```python
from build123d import *

# Parameters (mm, degrees)
SKETCH1_W                                = 68.4872
SKETCH1_H                                = 20.55
BOSS_EXTRUDE1_DEPTH                      = 28.732
SKETCH2_W                                = 55.7872
SKETCH2_H                                = 18.207
CUT_EXTRUDE1_DEPTH                       = 21.55
F_2_5_2_5_DIAMETER_HOLE1_AT_2_COUNT      = 2
F_2_5_2_5_DIAMETER_HOLE1_AT_2_PITCH      = 62.1372
F_3_2_3_2_DIAMETER_HOLE1_AT_2_COUNT      = 2
F_3_2_3_2_DIAMETER_HOLE1_AT_2_PITCH      = 62.1372
F_5_16_0_3125_DIAMETER_HOLE1_D           = 7.9375
F_5_16_0_3125_DIAMETER_HOLE1_CSINK_D     = 9.2075
F_5_16_0_3125_DIAMETER_HOLE1_CSINK_ANGLE = 90
F_1_8_0_125_DIAMETER_HOLE1_D             = 3.175
F_1_8_0_125_DIAMETER_HOLE1_DEPTH         = 9.53
F_1_8_0_125_DIAMETER_HOLE1_CSINK_D       = 3.81
F_1_8_0_125_DIAMETER_HOLE1_CSINK_ANGLE   = 90
F_1_8_0_125_DIAMETER_HOLE1_TIP           = 0.953866233


with BuildPart() as part:
    # Sketch1 → Boss-Extrude1 (new body)
    with BuildSketch(Plane(origin=(0, 0, 0), x_dir=(1, 0, 0), z_dir=(0, 1, 0))):
        with Locations((0, 10.275)):
            Rectangle(SKETCH1_W, SKETCH1_H)
    extrude(amount=BOSS_EXTRUDE1_DEPTH)

    # Sketch2 → Cut-Extrude1 (cut, through all)
    with BuildSketch(Plane.XY):
        with Locations((0, 19.6285)):
            Rectangle(SKETCH2_W, SKETCH2_H)
    extrude(amount=-CUT_EXTRUDE1_DEPTH, mode=Mode.SUBTRACT)

    # Sketch5 → Ø2.5 (2.5) Diameter Hole1 (revolve, cut)
    with BuildSketch(Plane(origin=(-31.0686, 21.5, 0), x_dir=(0, -1, 0), z_dir=(1, 0, 0))):
        Polygon((0, 0), (0, 20.55), (1.375, 20.55), (1.25, 20.425), (1.25, 0.125), (1.375, 0), align=None)
    f_2_5_2_5_diameter_hole1 = revolve(axis=Axis((-31.0686, 21.5, 6.35), (0, 0, -1)), mode=Mode.SUBTRACT)

    # Ø2.5 (2.5) Diameter Hole1 at 2: Ø2.5 (2.5) Diameter Hole1 ×2
    with Locations(*[(i * F_2_5_2_5_DIAMETER_HOLE1_AT_2_PITCH, 0, 0) for i in range(1, F_2_5_2_5_DIAMETER_HOLE1_AT_2_COUNT)]):
        add(f_2_5_2_5_diameter_hole1, mode=Mode.SUBTRACT)

    # Sketch8 → Ø3.2 (3.2) Diameter Hole1 (revolve, cut)
    with BuildSketch(Plane(origin=(-31.0686, 10.5, 0), x_dir=(0, -1, 0), z_dir=(1, 0, 0))):
        Polygon((0, 0), (0, 20.55), (1.75, 20.55), (1.6, 20.4), (1.6, 0.15), (1.75, 0), align=None)
    f_3_2_3_2_diameter_hole1 = revolve(axis=Axis((-31.0686, 10.5, 6.35), (0, 0, -1)), mode=Mode.SUBTRACT)

    # Ø3.2 (3.2) Diameter Hole1 at 2: Ø3.2 (3.2) Diameter Hole1 ×2
    with Locations(*[(i * F_3_2_3_2_DIAMETER_HOLE1_AT_2_PITCH, 0, 0) for i in range(1, F_3_2_3_2_DIAMETER_HOLE1_AT_2_COUNT)]):
        add(f_3_2_3_2_diameter_hole1, mode=Mode.SUBTRACT)

    # 5/16 (0.3125) Diameter Hole1 (through all)
    with Locations(Plane(origin=(0, 10.525, 0), x_dir=(-1, 0, 0), z_dir=(0, 1, 0))):
        with Locations((17.5, -11.55), (-17.5, -11.55)):
            CounterSinkHole(F_5_16_0_3125_DIAMETER_HOLE1_D / 2, F_5_16_0_3125_DIAMETER_HOLE1_CSINK_D / 2, counter_sink_angle=F_5_16_0_3125_DIAMETER_HOLE1_CSINK_ANGLE)

    # 1/8 (0.125) Diameter Hole1
    with Locations(Plane.XZ):
        with Locations((27.5, -11.55), (-27.5, -11.55)):
            CounterSinkHole(F_1_8_0_125_DIAMETER_HOLE1_D / 2, F_1_8_0_125_DIAMETER_HOLE1_CSINK_D / 2, depth=F_1_8_0_125_DIAMETER_HOLE1_DEPTH, counter_sink_angle=F_1_8_0_125_DIAMETER_HOLE1_CSINK_ANGLE)
            with Locations((0, 0, -(F_1_8_0_125_DIAMETER_HOLE1_DEPTH + F_1_8_0_125_DIAMETER_HOLE1_TIP / 2))):  # 118° drill point
                Cone(0, F_1_8_0_125_DIAMETER_HOLE1_D / 2, F_1_8_0_125_DIAMETER_HOLE1_TIP, mode=Mode.SUBTRACT)


solid = part.part
```
CAD build for the part. Positions are in the model's coordinates, mm. A direction names the side the tool comes from. Round coordinates to 2 decimals unless told otherwise and drop trailing zeros. Order: outer loops, then holes, each group sorted by start corner. A loop starts at its lowest first (then second) coordinate and runs counter-clockwise, first axis right, second up.
Q1. Wall check: L1, parallel to X at y = 6.25, z = -11.55; L2, parallel to Z at x = -17.5, y = 5.75; L3, parallel to Z at x = -27.5, y = 5.5. Give the ranges that are in metal, low to high.
Q2. Two-plate mould, pull along X, no slides. Class faces 1 (the flat face through (31, 28.732, -10)), 2 (the flat face through (34.244, 14, -10)), 3 (the flat face through (0, 10.525, -10)): pulls with the +X half, pulls with the -X half, needs draft (parallel to the pull), parting line crosses it, or undercut.
Q3. Slice it at D-D (z = -18.75). Write the cut outline in (x, y) (3 decimals), and give its area (3 significant figures).
Q4. Slice it at A-A (y = 21.5). Write the cut outline in (x, z) (3 decimals), and give its area (3 significant figures).
Q5. Slice it at B-B (x = -17.5). Write the cut outline in (y, z) (3 decimals), and give its area (3 significant figures).
Q6. Slice it at C-C (y = 3). State how many separate pieces and enclosed holes the cut face has, and give its area (3 significant figures).
Q7. Drop flat-ended pins along their axis: pin 1 (2 mm diameter, centred on x = 31.07, y = 21.5, fed in from -Z); pin 2 (9 mm diameter, centred on x = 17.5, z = -11.55, fed in from +Y); pin 3 (1.9 mm diameter, centred on x = 27.5, z = -11.55, fed in from -Y); pin 4 (6 mm diameter, centred on x = 2, z = -15, fed in from +Y) (3 decimals). Give the stop position or say it passes through.
Q8. Which spindle directions (+Z, -Z, +X, -X, +Y, -Y) get a long thin tool onto all of the face, cutting with end or side? Do faces 4 (the flat face through (-27.894, 20, -10)), 5 (the cylindrical face through (31.547, 20.345, -10.133)), 6 (the cylindrical face through (-29.014, 4.988, -11.073)). Say none if no direction does.
Results below:
1. L1: x = -34.24 to -29.09, -25.91 to -21.47, -13.53 to 13.53, 21.47 to 25.91, 29.09 to 34.24
1. L2: z = -20.55 to -15.52, -7.58 to 0
1. L3: z = -20.55 to -13.14, -9.96 to 0
2. face 1: needs draft
2. face 2: pulls with the +X half
2. face 3: undercut
3. outline: (-34.244, 0) - (34.244, 0) - (34.244, 28.732) - (27.894, 28.732) - (27.894, 10.525) - (-27.894, 10.525) - (-27.894, 28.732) - (-34.244, 28.732) - close; hole circle Ø3.2 at (-31.069, 10.5); hole circle Ø2.5 at (-31.069, 21.5); hole circle Ø3.2 at (31.069, 10.5); hole circle Ø2.5 at (31.069, 21.5)
3. area: 926 mm2
4. outline: (-34.244, -20.55) - (-32.444, -20.55) - (-32.319, -20.425) - (-32.319, -0.125) - (-32.444, 0) - (-34.244, 0) - close; (-29.819, -20.425) - (-29.694, -20.55) - (-27.894, -20.55) - (-27.894, 0) - (-29.694, 0) - (-29.819, -0.125) - close; (27.894, -20.55) - (29.694, -20.55) - (29.819, -20.425) - (29.819, -0.125) - (29.694, 0) - (27.894, 0) - close; (32.319, -20.425) - (32.444, -20.55) - (34.244, -20.55) - (34.244, 0) - (32.444, 0) - (32.319, -0.125) - close
4. area: 158 mm2
5. outline: (0, -20.55) - (10.525, -20.55) - (10.525, -16.154) - (9.89, -15.519) - (0, -15.519) - close; (0, -7.581) - (9.89, -7.581) - (10.525, -6.946) - (10.525, 0) - (0, 0) - close
5. area: 132 mm2
6. separate pieces: 1
6. enclosed holes: 4
6. area: 1,290 mm2
7. pin 1: passes through
7. pin 2: stops at y = 10.42
7. pin 3: stops at y = 9.91
7. pin 4: stops at y = 10.525
8. face 4: +Z, -Z, +Y
8. face 5: +Z, -Z
8. face 6: -Y
